Answer from the drawing. Dimensions are ordinates in mm from the lowest x, y and z of the part. Give positions to 0.01 mm unless a question says otherwise; leave off trailing zeros. Loops run counter-clockwise (first coordinate to the right, second up) from the corner with the lowest first, then second, coordinate; pieces in that order, holes last.
Item 1: Section C-C, the plane x = 65 is taken. Give the vertices of the cut face in (y, z) (1 decimal).
Item 2: The mould has two halves that part along X. Classify the marked faces 1, 2 and 3: pulls with the +X half, pulls with the -X half, needs draft (parallel to the pull), parting line crosses it, or undercut.
Item 3: Section A-A, the plane z = 7.5 is taken. Give the vertices of the cut face in (x, y) (1 decimal).
Item 4: This flat-tipped pin is pushed along its axis until it touches: pin 1 Ø1 at (x, y) = (61, 1.5) entering from -Z. Where does it stop, or does it pass through?
Item 5: Consider line 1 along Z through (x, y) = (87.5, 2.5) (1 decimal); line 2 along X through (y, z) = (3.5, 7.5) (1 decimal); line 3 along X through (y, z) = (4.75, 26). Determine where each line is inside the solid, lowest interval first.
Item 6: Section D-D, the plane y = 4.25 is taken. Give the number of separate pieces and of enclosed holes in the cut face, and give its area (3 significant figures).
Item 7: Section B-B, the plane z = 34 is taken. Give the vertices of the cut face in (x, y), and give its area (3 significant figures).
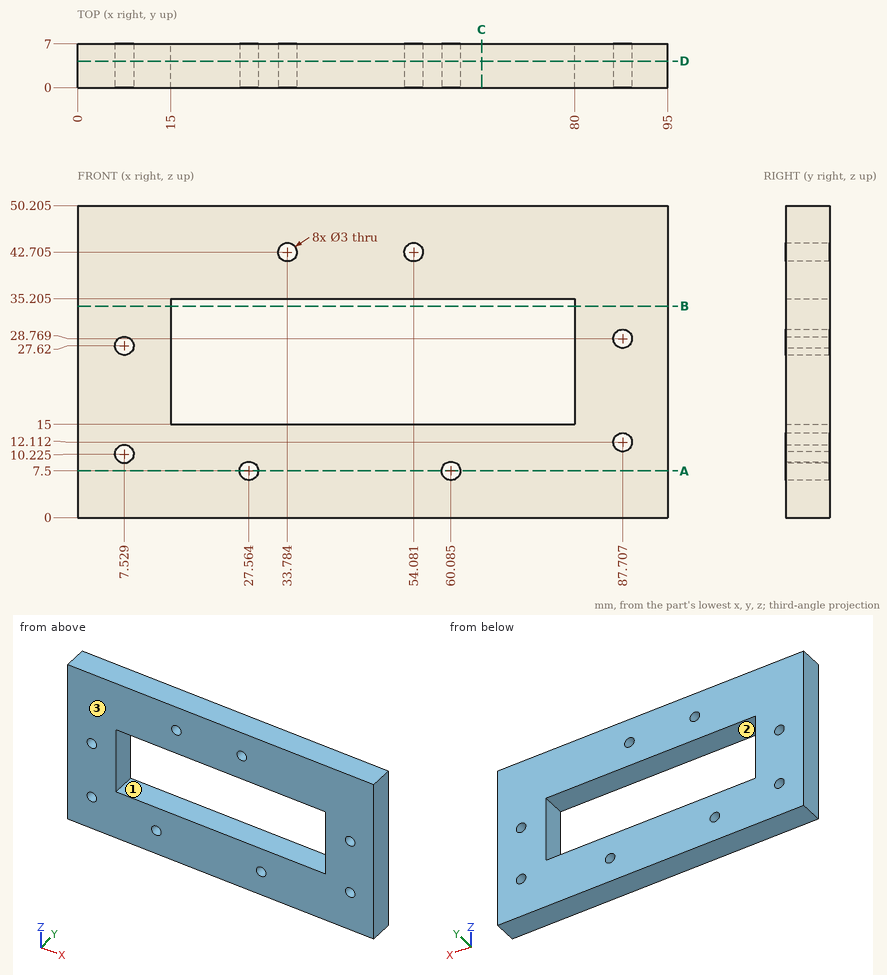
Worked answers:
1. outline: (0, 0) - (7, 0) - (7, 15) - (0, 15) - close; (0, 35.2) - (7, 35.2) - (7, 50.2) - (0, 50.2) - close
2. face 1: undercut
2. face 2: undercut
2. face 3: needs draft
3. outline: (0, 0) - (26.1, 0) - (26.1, 7) - (0, 7) - close; (29.1, 0) - (58.6, 0) - (58.6, 7) - (29.1, 7) - close; (61.6, 0) - (95, 0) - (95, 7) - (61.6, 7) - close
4. pin 1: stops at z = 0
5. line 1: z = 0 to 10.6, 13.6 to 27.3, 30.3 to 50.2
5. line 2: x = 0 to 26.1, 29.1 to 58.6, 61.6 to 95
5. line 3: x = 0 to 15, 80 to 95
6. separate pieces: 1
6. enclosed holes: 9
6. area: 3,400 mm2
7. outline: (0, 0) - (15, 0) - (15, 7) - (0, 7) - close; (80, 0) - (95, 0) - (95, 7) - (80, 7) - close
7. area: 210 mm2
